Read the model definition and answer for the solid it produces. Units are mm, in the model's axes. Give positions to 0.01 mm unless a question says otherwise; leave off trailing zeros. Loops run counter-clockwise (first coordinate to the right, second up) from the corner with the lowest first, then second, coordinate; pieces in that order, holes last.
(1) Each of these flat-tipped pins is pushed along its axis until it touches: P1, Ø1, axis at y = 0, z = -31.5, coming from the -X side; P2, Ø1, axis at x = -49.5, y = 0.5, coming from the +Z side; P3, Ø1, axis at x = 22, y = -0.5, coming from the +Z side; P4, Ø5.5, axis at x = -50.7, z = 0, coming from the -Y side. Where does it stop, or does it pass through?
(2) Find section C-C, the plane z = 28. Write down the section's boundary in (x, y), then the cut area to 3 significant figures.
(3) Find section A-A, the plane x = 0. Write down the section's boundary in (y, z), then the cut area to 3 significant figures.
(4) Find section D-D, the plane y = 0.25. State how many separate pieces and enclosed holes the cut face has, then the cut area to 3 significant figures.
(5) Find section B-B, the plane z = 0. Write down the section's boundary in (x, y).
(6) Straight lines are drawn through the part: probe 1 along X at (y, z) = (-0.75, -3); probe 2 along X at (y, z) = (-0.5, 50.7). For each, find the intervals that lie inside material, in ascending order.
(7) Determine the mould class of faces 1 (the face through (-0.14, 0.01, -57.05)), 2 (the face through (57.05, 0.01, -0.14)), 3 (the face through (-42.551, 0.014, -8.174)), 4 (the face through (47.605, 0.014, -1.283)) for opening direction X: pulls with the +X half, pulls with the -X half, needs draft (parallel to the pull), parting line crosses it, or undercut.
```python
from build123d import *

# Parameters (mm, degrees)
SKETCH1_R           = 41
SKETCH1_R_2         = 36
BOSS_EXTRUDE1_DEPTH = 1
SKETCH2_R           = 3.35
BOSS_EXTRUDE2_DEPTH = 2
CIRPATTERN1_COUNT   = 4


with BuildPart() as part:
    # Sketch1 → Boss-Extrude1 (new, symmetric)
    with BuildSketch(Plane(origin=(0, 0, 0), x_dir=(1, 0, 0), z_dir=(0, 1, 0))):
        with Locations(Location((0, 0, 0), (0, 0, 270))):
            Circle(SKETCH1_R)
        with Locations(Location((0, 0, 0), (0, 0, 270))):
            Circle(SKETCH1_R_2, mode=Mode.SUBTRACT)
    extrude(amount=BOSS_EXTRUDE1_DEPTH, both=True)

    # Sketch2 → Boss-Extrude2 (add)
    with BuildSketch(Plane(origin=(0, 1, 0), x_dir=(1, 0, 0), z_dir=(0, 1, 0))):
        with BuildLine():
            Line((-6.35, 48.308151486), (-6.35, 50.7))
            ThreePointArc((-6.35, 50.7), (0, 57.05), (6.35, 50.7))
            Line((6.35, 50.7), (6.35, 48.308151486))
            ThreePointArc((6.35, 48.308151486), (8.224151628, 42.479722175), (13.144117647, 38.83596492))
            ThreePointArc((13.144117647, 38.83596492), (0, 41), (-13.144117647, 38.83596492))
            ThreePointArc((-13.144117647, 38.83596492), (-8.224151628, 42.479722175), (-6.35, 48.308151486))
        make_face()
        with Locations(Location((0, 50.7, 0), (0, 0, 270))):
            Circle(SKETCH2_R, mode=Mode.SUBTRACT)
    boss_extrude2 = extrude(amount=-BOSS_EXTRUDE2_DEPTH)

    # CirPattern1: Boss-Extrude2 ×4 about axis
    cirpattern1_axis = Axis((0, 0, 0), (0, 1, 0))
    for i in range(1, CIRPATTERN1_COUNT):
        add(boss_extrude2.rotate(cirpattern1_axis, i * 360 / CIRPATTERN1_COUNT))


solid = part.part
```
Entries:
1. P1: stops at x = -26.83
1. P2: stops at z = 6.35
1. P3: stops at z = 34.91
1. P4: passes through
2. outline: (-29.95, -1) - (-22.63, -1) - (-22.63, 1) - (-29.95, 1) - close; (22.63, -1) - (29.95, -1) - (29.95, 1) - (22.63, 1) - close
2. area: 29.3 mm2
3. outline: (-1, -57.05) - (1, -57.05) - (1, -54.05) - (-1, -54.05) - close; (-1, -47.35) - (1, -47.35) - (1, -36) - (-1, -36) - close; (-1, 36) - (1, 36) - (1, 47.35) - (-1, 47.35) - close; (-1, 54.05) - (1, 54.05) - (1, 57.05) - (-1, 57.05) - close
3. area: 57.4 mm2
4. separate pieces: 1
4. enclosed holes: 5
4. area: 1,910 mm2
5. outline: (-57.05, -1) - (-54.05, -1) - (-54.05, 1) - (-57.05, 1) - close; (-47.35, -1) - (-36, -1) - (-36, 1) - (-47.35, 1) - close; (36, -1) - (47.35, -1) - (47.35, 1) - (36, 1) - close; (54.05, -1) - (57.05, -1) - (57.05, 1) - (54.05, 1) - close
6. probe 1: x = -56.3 to -52.19, -49.21 to -35.87, 35.87 to 49.21, 52.19 to 56.3
6. probe 2: x = -6.35 to -3.35, 3.35 to 6.35
7. face 1: parting line crosses it
7. face 2: pulls with the +X half
7. face 3: pulls with the -X half
7. face 4: undercut
